Work out the finished part from the listing and answer in its coordinate system (mm). A direction names the side the tool comes from. Give positions to 0.01 mm unless a question says otherwise; leave off trailing zeros. Loops run counter-clockwise (first coordinate to the right, second up) from the corner with the lowest first, then second, coordinate; pieces in that order, holes last.
```python
from build123d import *

# Parameters (mm, degrees)
SKETCH1_R           = 2.1
BOSS_EXTRUDE1_DEPTH = 4
SKETCH2_W           = 4
SKETCH2_H           = 79.366859707
BOSS_EXTRUDE2_DEPTH = 36
SKETCH3_W           = 16.795845367
SKETCH3_H           = 36
CUT_EXTRUDE1_DEPTH  = 20
SKETCH4_W           = 16
SKETCH4_H           = 4
BOSS_EXTRUDE3_DEPTH = 36
CUT_EXTRUDE2_DEPTH  = 20
BOSS_EXTRUDE4_DEPTH = 3
CUT_EXTRUDE3_DEPTH  = 3
SKETCH9_W           = 24
SKETCH9_H           = 16
CUT_EXTRUDE5_DEPTH  = 4
FILLET1_R           = 2
FILLET2_R           = 2
FILLET3_START       = -20
FILLET3_DEPTH       = 57.57101424
FILLET3_START_2     = 35.417415549
FILLET3_2_DEPTH     = 8.582584451
FILLET3_START_3     = 39
FILLET3_4_DEPTH     = 5


with BuildPart() as part:
    # Sketch1 → Boss-Extrude1 (new body)
    with BuildSketch(Plane(origin=(0, 0, 0), x_dir=(1, 0, 0), z_dir=(0, 1, 0))):
        with BuildLine():
            Line((-12, 20), (12, 20))
            ThreePointArc((12, 20), (14.828427125, 18.828427125), (16, 16))
            Line((16, 16), (16, -16))
            Line((16, -16), (16, -26.57101434))
            Line((16, -26.57101434), (-16, -26.57101434))
            Line((-16, -26.57101434), (-20, -26.57101434))
            Line((-20, -26.57101434), (-20, 20))
            Line((-20, 20), (-12, 20))
        make_face()
        with Locations(Location((-12, 16, 0), (0, 0, 270))):
            Circle(SKETCH1_R, mode=Mode.SUBTRACT)
        with Locations(Location((12, 16, 0), (0, 0, 270))):
            Circle(SKETCH1_R, mode=Mode.SUBTRACT)
        with Locations(Location((12, -16, 0), (0, 0, 270))):
            Circle(SKETCH1_R, mode=Mode.SUBTRACT)
        with Locations(Location((-12, -16, 0), (0, 0, 270))):
            Circle(SKETCH1_R, mode=Mode.SUBTRACT)
        with BuildLine():
            Line((-8, 16), (8, 16))
            ThreePointArc((8, 16), (9.171572875, 13.171572875), (12, 12))
            Line((12, 12), (12, -12))
            ThreePointArc((12, -12), (9.171572875, -13.171572875), (8, -16))
            Line((8, -16), (-8, -16))
            ThreePointArc((-8, -16), (-9.171572875, -13.171572875), (-12, -12))
            Line((-12, -12), (-12, 12))
            ThreePointArc((-12, 12), (-9.171572875, 13.171572875), (-8, 16))
        make_face(mode=Mode.SUBTRACT)
    extrude(amount=BOSS_EXTRUDE1_DEPTH)

    # Sketch2 → Boss-Extrude2 (add)
    with BuildSketch(Plane(origin=(0, 4, 0), x_dir=(1, 0, 0), z_dir=(0, 1, 0))):
        with Locations((-18, -19.683429854)):
            Rectangle(SKETCH2_W, SKETCH2_H)
    extrude(amount=BOSS_EXTRUDE2_DEPTH)

    # Sketch3 → Cut-Extrude1 (cut)
    with BuildSketch(Plane.ZY.offset(20)):
        Polygon((-20, 4), (33.57101434, 40), (-20, 40), align=None)
        with Locations((50.968937024, 22)):
            Rectangle(SKETCH3_W, SKETCH3_H)
    extrude(amount=-CUT_EXTRUDE1_DEPTH, mode=Mode.SUBTRACT)

    # Sketch4 → Boss-Extrude3 (add)
    with BuildSketch(Plane.ZY.offset(20)):
        with Locations((34.57101434, 2)):
            Rectangle(SKETCH4_W, SKETCH4_H)
    extrude(amount=-BOSS_EXTRUDE3_DEPTH)

    # Sketch5 → Cut-Extrude2 (cut)
    with BuildSketch(Plane.ZY.offset(20)):
        Polygon((33.57101434, 34), (33.57101434, 9), (-3.42898566, 9), align=None)
    extrude(amount=-CUT_EXTRUDE2_DEPTH, mode=Mode.SUBTRACT)

    # Sketch6 → Boss-Extrude4 (add)
    with BuildSketch(Plane.XY.offset(42.57101434)):
        Polygon((-16, 40), (-16, 4), (16, 4), align=None)
    extrude(amount=-BOSS_EXTRUDE4_DEPTH)

    # Sketch7 → Cut-Extrude3 (cut)
    with BuildSketch(Plane(origin=(0, 0, 39.57101434), x_dir=(-1, 0, 0), z_dir=(0, 0, -1))):
        Polygon((13.171572875, 6.828427125), (13.171572875, 30.828427125), (-8.598354134, 6.828427125), align=None)
    extrude(amount=-CUT_EXTRUDE3_DEPTH, mode=Mode.SUBTRACT)

    # Sketch9 → Cut-Extrude5 (cut)
    with BuildSketch(Plane.XZ):
        with Locations((0, 29.1)):
            Rectangle(SKETCH9_W, SKETCH9_H)
    extrude(amount=-CUT_EXTRUDE5_DEPTH, mode=Mode.SUBTRACT)

    # Fillet1
    fillet1_edges = [part.edges().sort_by_distance(p)[0] for p in [
        (-18, 9, -3.42898566),
        (-18, 34, 33.57101434),
        (-18, 9, 33.57101434),
        (-13.171572875, 6.828427125, 41.07101434),
        (8.598354134, 6.828427125, 41.07101434),
        (-13.171572875, 30.828427125, 41.07101434),
        (12, 2, 37.1),
        (12, 2, 21.1),
        (-12, 2, 21.1),
        (-12, 2, 37.1),
        (-8, 2, -16),
        (-12, 2, -12),
        (-12, 2, 12),
        (-8, 2, 16),
        (8, 2, 16),
        (12, 2, 12),
        (12, 2, -12),
        (8, 2, -16),
    ]]
    fillet(fillet1_edges, radius=FILLET1_R)

    # Fillet2
    fillet2_edges = [part.edges().sort_by_distance(p)[0] for p in [
        (-20, 0, 11.28550717),
        (0, 4, 39.57101434),
        (-16, 22, 39.57101434),
        (-20, 40, 38.07101434),
    ]]
    fillet(fillet2_edges, radius=FILLET2_R)

    # Fillet3: read off the stored shape, not the designer's step
    # Fillet3 outline → Fillet3 (cut)
    with BuildSketch(Plane.XY.offset(FILLET3_START)):
        with BuildLine():
            ThreePointArc((-18, 40), (-16.585786438, 39.414213562), (-16, 38))
            Line((-16, 38), (-16, 40))
            Line((-16, 40), (-18, 40))
        make_face()
    extrude(amount=FILLET3_DEPTH, mode=Mode.SUBTRACT)

    # Fillet3 2 outline → Fillet3 2 (cut)
    with BuildSketch(Plane.XY.offset(FILLET3_START_2)):
        with BuildLine():
            Line((-16, 40), (-16.898132129, 40))
            ThreePointArc((-16.898132129, 40), (-16.43660977, 39.946020841), (-16, 39.786997113))
            Line((-16, 39.786997113), (-16, 40))
        make_face()
    extrude(amount=FILLET3_2_DEPTH, mode=Mode.SUBTRACT)

    # Fillet3 3 outline → Fillet3 3 (revolve, cut)
    with BuildSketch(Plane(origin=(-14, 0, 37.57101434), x_dir=(1, 0, 0), z_dir=(0, 0, 1))):
        with BuildLine():
            Line((2, 40), (2, 38))
            ThreePointArc((2, 38), (2.585786438, 39.414213562), (4, 40))
            Line((4, 40), (2, 40))
        make_face()
    revolve(axis=Axis((-14, 0, 37.57101434), (0, 1, 0)), mode=Mode.SUBTRACT)

    # Fillet3 4 outline → Fillet3 4 (cut)
    with BuildSketch(Plane.XY.offset(FILLET3_START_3)):
        with BuildLine():
            ThreePointArc((-16, 39.786997113), (-15.679913732, 39.586172734), (-15.403313491, 39.328727678))
            Line((-15.403313491, 39.328727678), (-16, 40))
            Line((-16, 40), (-16, 39.786997113))
        make_face()
    extrude(amount=FILLET3_4_DEPTH, mode=Mode.SUBTRACT)


solid = part.part
```
Q1. Section D-D on z = -13 is taken. Give the vertices of the cut face in (x, y), plus the area to 3 significant figures.
Q2. Section B-B on z = 32.5 is taken. Give the vertices of the cut face in (x, y), plus the area to 3 significant figures.
Q3. Which of the six approach directions +Z, -Z, +X, -X, +Y, -Y give full straight-line access (tool end or side, diameter ignored) to faces 1 (the face through (-2.17, 18.7, 41.05)), 2 (the face through (-17.97, 10.45, 1.18)), 3 (the face through (-7.512, 2.028, 15.623))?
Q4. Determine the mould class of faces 4 (the face through (-17.972, 32.015, 32.482)), 5 (the face through (0.518, 21.417, 41.217)), 6 (the face through (14.082, 1.972, 15.727)), 7 (the face through (-3, 6.828, 41)) for opening direction X: +X half, -X half, draft (parallel to the pull), parting line (faces both ways), or undercut.
Q5. Section C-C on y = 31 is taken. Give the vertices of the cut face in (x, z), plus the area to 3 significant figures.
Q6. Given pin 1 (2.5 mm diameter, centred on x = -1.5, z = 41.5, fed in from +Y); pin 2 (14 mm diameter, centred on x = 2, y = 18, fed in from -Z); pin 3 (2 mm diameter, centred on x = 11.5, z = -12.5, fed in from +Y); pin 4 (3 mm diameter, centred on x = -7.5, z = 35, fed in from +Y), each flat-ended and moving along its own axis, determine where each tip first touches the part or whether it passes through.
Q7. Section A-A on x = -3 is taken. Give the vertices of the cut face in (y, z) (3 decimals), plus the area to 3 significant figures.
Q8. Consider line 1 along Z through (x, y) = (2.5, 2); line 2 along Y through (x, z) = (-15, 12); line 3 along X through (y, z) = (14, 36). Determine where each line is inside the solid, lowest interval first.
Check result:
1. outline: (-20, 2) arc R2 ccw to (-18, 0) - (-9.35, 0) - (-9.35, 4) - (-16, 4) - (-16, 8.7) - (-20, 8.7) - close; (9.35, 0) - (16, 0) - (16, 4) - (9.35, 4) - close
1. area: 87.1 mm2
2. outline: (-20, 2) arc R2 ccw to (-18, 0) - (-12, 0) - (-12, 4) - (-16, 4) - (-16, 9.23) - (-20, 9.23) - close; (-20, 32.01) - (-16, 32.01) - (-16, 38) arc R2 ccw to (-16.46, 39.28) - (-19.54, 39.28) arc R2 ccw to (-20, 38) - close; (12, 0) - (16, 0) - (16, 4) - (12, 4) - close
2. area: 96.8 mm2
3. face 1: +Z, -Z
3. face 2: +X, -X
3. face 3: +Y, -Y
4. face 4: draft
4. face 5: +X half
4. face 6: undercut
4. face 7: undercut
5. outline: (-20, 20.18) - (-16, 20.18) - (-16, 29.13) - (-20, 29.13) - close; (-20, 33.42) - (-16, 33.42) - (-16, 37.57) arc R2 cw to (-14, 39.57) - (-8, 39.57) - (-8, 42.57) - (-20, 42.57) - close
5. area: 97.3 mm2
6. pin 1: stops at y = 25.09
6. pin 2: stops at z = 39.57
6. pin 3: stops at y = 4
6. pin 4: passes through
7. outline: (0, -20) - (4, -20) - (4, -16) - (0, -16) - close; (0, 16) - (4, 16) - (4, 21.1) - (0, 21.1) - close; (0, 37.1) - (4, 37.1) - (4, 37.571) arc R2 cw to (6, 39.571) - (6.828, 39.571) - (6.828, 42.571) - (0, 42.571) - close; (19.615, 39.571) - (25.375, 39.571) - (25.375, 42.571) - (19.615, 42.571) - close
7. area: 84.9 mm2
8. line 1: z = -20 to -16, 16 to 21.1, 37.1 to 42.57
8. line 2: y = 0 to 4
8. line 3: x = -20 to -16
